```python
from build123d import *

# Parameters (mm, degrees)
CYLINDER002_R       = 2.1
CYLINDER002_DEPTH   = 10
CYLINDER001_R       = 2.1
CYLINDER001_DEPTH   = 10
BOX_W               = 7
BOX_H               = 8
BOX_DEPTH           = 17
BOX_PLACEMENT_ANGLE = 9


with BuildPart() as cylinder002:
    # Cylinder002 → Cylinder002 (new body)
    with BuildSketch(Plane(origin=(23, 39.6, 42.2), x_dir=(0, 0, -1), z_dir=(1, 0, 0))):
        Circle(CYLINDER002_R)
    extrude(amount=CYLINDER002_DEPTH)


with BuildPart() as fusion:
    # Cylinder001 → Cylinder001 (new body)
    with BuildSketch(Plane(origin=(23, 38, 32.3), x_dir=(0, 0, -1), z_dir=(1, 0, 0))):
        Circle(CYLINDER001_R)
    extrude(amount=CYLINDER001_DEPTH)

    # Fusion: union Cylinder002
    add(cylinder002.part)


with BuildPart() as fusion_1:
    # Fusion placement: moved
    add(fusion.part.moved(Location((-1, 0, 0))))


with BuildPart() as cut001:
    # Box → Box (new body)
    with BuildSketch(Plane.XY):
        with Locations((3.5, 4)):
            Rectangle(BOX_W, BOX_H)
    extrude(amount=BOX_DEPTH)


with BuildPart() as cut001_1:
    # Box placement: moved
    add(cut001.part.moved(Location((20.2, 33, 29.5))).rotate(Axis((20.2, 33, 29.5), (-1, 0, 0)), BOX_PLACEMENT_ANGLE))

    # Cut001: cut Fusion
    add(fusion_1.part, mode=Mode.SUBTRACT)


solid = cut001_1.part
```
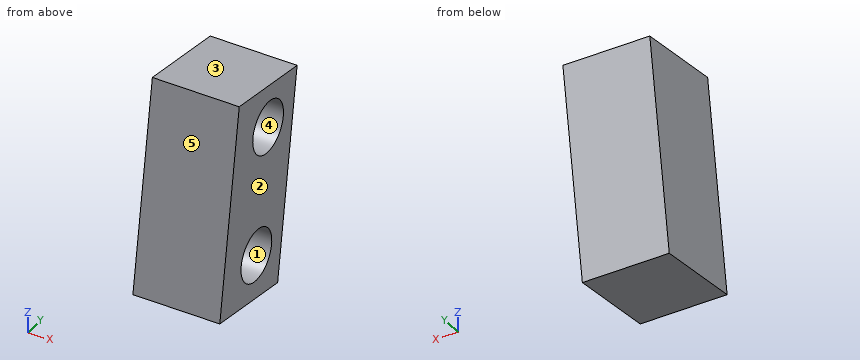
Can you work these out from the model? Positions are in its coordinate system, mm. Face numbers are marked on the shaded views. A direction names the side the tool comes from. Coordinates: 2 decimals unless noted, no trailing zeros. Loops run counter-clockwise (first coordinate to the right, second up) from the corner with the lowest first, then second, coordinate; pieces in that order, holes last. Notation, with made-up numbers: (38, -7.5) -> (74, -7.5) arc R23 ccw to (74, 9.5) -> close; hole circle Ø3 at (-17.5, -24.75). An arc over 180 degrees is marked (long way). Put each result on its own line as item: value. Start each with the question number.
Q1. For the marked faces 4 and 5, which set-ups out of +Z, -Z, +X, -X, +Y, -Y let a thin tool reach every point of the face, with its end or its side?
Q2. I want a section at C-C (y = 41.25). Write out the boundary of the cut face in (x, z), plus the area to 3 significant figures.
Q3. If I drill on line 1 (Z direction, x = 25.85, y = 39.6); line 2 (Z direction, x = 25.3, y = 38); line 3 (Z direction, x = 24.5, y = 40.5), over which ranges is the centre line in solid material (lowest first)? Write a range as [from, to].
Q4. Thinking about a two-plate mould opening in Y: for the marked faces 1, 2 and 3, which applies, pulls with the +Y half, pulls with the -Y half, needs draft (parallel to the pull), parting line crosses it, or undercut?
Q5. I'm going to push flat-ended pins straight in: P1, Ø3.5, axis at y = 39.6, z = 42.2, coming from the +X side; P2, Ø4, axis at x = 21, z = 37, coming from the +Y side; P3, Ø1, axis at x = 22.5, y = 37.5, coming from the +Z side. Where does each tip first touch, or does it pass through?
Q6. I want a section at D-D (x = 21.5). Write out the boundary of the cut face in (y, z), plus the area to 3 significant figures.
Q7. I want a section at A-A (x = 22.5). Write out the boundary of the cut face in (y, z), plus the area to 3 significant figures.
Q8. I want a section at B-B (z = 32.3). Write out the boundary of the cut face in (x, y), plus the area to 3 significant figures.
Taken from the geometry:
1. face 4: +X
1. face 5: +Z, +X, -X, -Y
2. outline: (20.2, 30.45) -> (27.2, 30.45) -> (27.2, 40.9) -> (22, 40.9) -> (22, 43.5) -> (27.2, 43.5) -> (27.2, 45.41) -> (20.2, 45.41) -> close
2. area: 91.2 mm2
3. line 1: z = [28.45, 30.94], [33.66, 40.1], [44.3, 45.67]
3. line 2: z = [28.71, 30.2], [34.4, 40.84], [43.56, 45.92]
3. line 3: z = [28.31, 40.3], [44.1, 45.52]
4. face 1: undercut
4. face 2: needs draft
4. face 3: pulls with the +Y half
5. P1: stops at x = 22
5. P2: stops at y = 42.6
5. P3: stops at z = 46.08
6. outline: (33, 29.5) -> (40.9, 28.25) -> (43.56, 45.04) -> (35.66, 46.29) -> close
6. area: 136 mm2
7. outline: (33, 29.5) -> (40.9, 28.25) -> (43.56, 45.04) -> (35.66, 46.29) -> close; hole circle Ø4.2 at (38, 32.3); hole circle Ø4.2 at (39.6, 42.2)
7. area: 108 mm2
8. outline: (20.2, 33.44) -> (27.2, 33.44) -> (27.2, 35.9) -> (22, 35.9) -> (22, 40.1) -> (27.2, 40.1) -> (27.2, 41.54) -> (20.2, 41.54) -> close
8. area: 34.9 mm2
